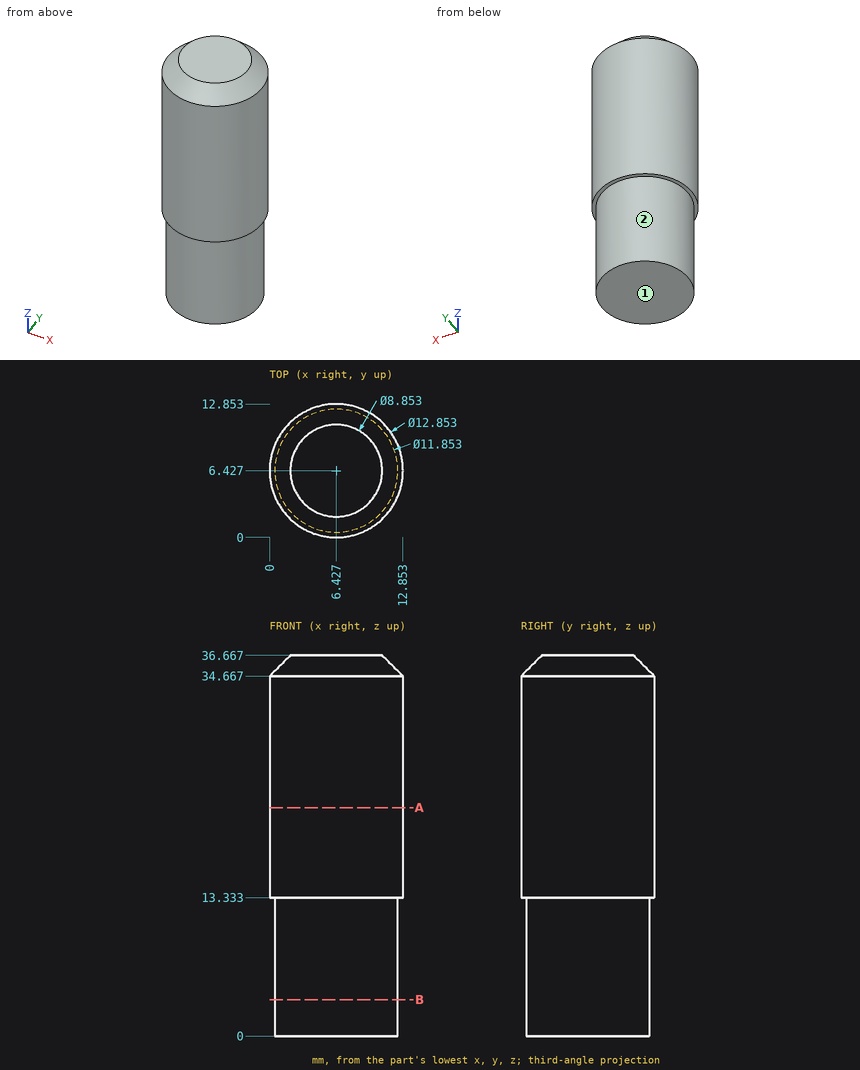
Verification items for this drawing (mm, ordinates from the low corner). Give positions to 0.01 mm unless a question says otherwise; leave off trailing zeros. Write each loop counter-clockwise with the first axis right and the second up, starting at its lowest first coordinate (ties: lowest second). Pieces come first, ordered by that corner, then holes. Notation, with made-up numbers: (63.5, -24) -> (78.5, -24) arc R8 cw to (78.5, -19) -> close; hole circle Ø5 at (-26.5, 39). An arc over 180 degrees is marked (long way). Use CSV: the item, a comma, the result in double quotes.
(1) Sectioned sample at A-A (z = 22). Record the cut outline in (x, y).
Derived:
outline,"circle Ø12.85 at (6.43, 6.43)"
(2) Go/stop test with a flat-tipped pin: pin 1 (1.5 mm diameter, centred on y = 11.5, z = 15.5, fed in from -X). Record where the tip stops, or that it passes through.
Derived:
pin 1,"stops at x = 1.67"
(3) Material ranges on L1, parallel to Y at x = 6.25, z = 11; L2, parallel to Y at x = 6.25, z = 27; L3, parallel to X at y = 2, z = 10.5 (1 decimal), recorded low to high.
Derived:
L1,"y = 0.5 to 12.35"
L2,"y = 0 to 12.85"
L3,"x = 2.5 to 10.4"
(4) Sectioned sample at B-B (z = 3.5). Record the cut outline in (x, y), plus the area to 3 significant figures.
Derived:
outline,"circle Ø11.85 at (6.43, 6.43)"
area,"110 mm^2"
(5) Release check for a two-part mould opening along Y. For the marked faces 1 and 2 record: +Y half, -Y half, draft (parallel to the pull), parting line (faces both ways), or undercut.
Derived:
face 1,"draft"
face 2,"parting line"
